from build123d import *

# Parameters (mm, degrees)
BOSS_EXTRUDE1_DEPTH = 6
FILLET1_R           = 10


with BuildPart() as part:
    # Sketch1 → Boss-Extrude1 (new body)
    with BuildSketch(Plane.XY):
        Polygon((0, 0), (24, 0), (24, -3), (34, -3), (34, 0), (154, 0), (154, -3), (164, -3), (164, 0), (193, 0), (179, 10), (29, 10), align=None)
        with BuildLine():
            Line((53.5, 7), (60.5, 7))
            ThreePointArc((60.5, 7), (60.853553391, 6.853553391), (61, 6.5))
            Line((61, 6.5), (61, 3.5))
            ThreePointArc((61, 3.5), (60.853553391, 3.146446609), (60.5, 3))
            Line((60.5, 3), (53.5, 3))
            ThreePointArc((53.5, 3), (53.146446609, 3.146446609), (53, 3.5))
            Line((53, 3.5), (53, 6.5))
            ThreePointArc((53, 6.5), (53.146446609, 6.853553391), (53.5, 7))
        make_face(mode=Mode.SUBTRACT)
        with BuildLine():
            Line((37.5, 7), (44.5, 7))
            ThreePointArc((44.5, 7), (44.853553391, 6.853553391), (45, 6.5))
            Line((45, 6.5), (45, 3.5))
            ThreePointArc((45, 3.5), (44.853553391, 3.146446609), (44.5, 3))
            Line((44.5, 3), (37.5, 3))
            ThreePointArc((37.5, 3), (37.146446609, 3.146446609), (37, 3.5))
            Line((37, 3.5), (37, 6.5))
            ThreePointArc((37, 6.5), (37.146446609, 6.853553391), (37.5, 7))
        make_face(mode=Mode.SUBTRACT)
        with BuildLine():
            Line((69.5, 7), (76.5, 7))
            ThreePointArc((76.5, 7), (76.853553391, 6.853553391), (77, 6.5))
            Line((77, 6.5), (77, 3.5))
            ThreePointArc((77, 3.5), (76.853553391, 3.146446609), (76.5, 3))
            Line((76.5, 3), (69.5, 3))
            ThreePointArc((69.5, 3), (69.146446609, 3.146446609), (69, 3.5))
            Line((69, 3.5), (69, 6.5))
            ThreePointArc((69, 6.5), (69.146446609, 6.853553391), (69.5, 7))
        make_face(mode=Mode.SUBTRACT)
        with BuildLine():
            Line((85.5, 7), (92.5, 7))
            ThreePointArc((92.5, 7), (92.853553391, 6.853553391), (93, 6.5))
            Line((93, 6.5), (93, 3.5))
            ThreePointArc((93, 3.5), (92.853553391, 3.146446609), (92.5, 3))
            Line((92.5, 3), (85.5, 3))
            ThreePointArc((85.5, 3), (85.146446609, 3.146446609), (85, 3.5))
            Line((85, 3.5), (85, 6.5))
            ThreePointArc((85, 6.5), (85.146446609, 6.853553391), (85.5, 7))
        make_face(mode=Mode.SUBTRACT)
        with BuildLine():
            Line((101.5, 7), (108.5, 7))
            ThreePointArc((108.5, 7), (108.853553391, 6.853553391), (109, 6.5))
            Line((109, 6.5), (109, 3.5))
            ThreePointArc((109, 3.5), (108.853553391, 3.146446609), (108.5, 3))
            Line((108.5, 3), (101.5, 3))
            ThreePointArc((101.5, 3), (101.146446609, 3.146446609), (101, 3.5))
            Line((101, 3.5), (101, 6.5))
            ThreePointArc((101, 6.5), (101.146446609, 6.853553391), (101.5, 7))
        make_face(mode=Mode.SUBTRACT)
        with BuildLine():
            Line((117.5, 7), (124.5, 7))
            ThreePointArc((124.5, 7), (124.853553391, 6.853553391), (125, 6.5))
            Line((125, 6.5), (125, 3.5))
            ThreePointArc((125, 3.5), (124.853553391, 3.146446609), (124.5, 3))
            Line((124.5, 3), (117.5, 3))
            ThreePointArc((117.5, 3), (117.146446609, 3.146446609), (117, 3.5))
            Line((117, 3.5), (117, 6.5))
            ThreePointArc((117, 6.5), (117.146446609, 6.853553391), (117.5, 7))
        make_face(mode=Mode.SUBTRACT)
        with BuildLine():
            Line((133.5, 7), (140.5, 7))
            ThreePointArc((140.5, 7), (140.853553391, 6.853553391), (141, 6.5))
            Line((141, 6.5), (141, 3.5))
            ThreePointArc((141, 3.5), (140.853553391, 3.146446609), (140.5, 3))
            Line((140.5, 3), (133.5, 3))
            ThreePointArc((133.5, 3), (133.146446609, 3.146446609), (133, 3.5))
            Line((133, 3.5), (133, 6.5))
            ThreePointArc((133, 6.5), (133.146446609, 6.853553391), (133.5, 7))
        make_face(mode=Mode.SUBTRACT)
        with BuildLine():
            Line((149.5, 7), (156.5, 7))
            ThreePointArc((156.5, 7), (156.853553391, 6.853553391), (157, 6.5))
            Line((157, 6.5), (157, 3.5))
            ThreePointArc((157, 3.5), (156.853553391, 3.146446609), (156.5, 3))
            Line((156.5, 3), (149.5, 3))
            ThreePointArc((149.5, 3), (149.146446609, 3.146446609), (149, 3.5))
            Line((149, 3.5), (149, 6.5))
            ThreePointArc((149, 6.5), (149.146446609, 6.853553391), (149.5, 7))
        make_face(mode=Mode.SUBTRACT)
        with BuildLine():
            Line((165.5, 7), (172.5, 7))
            ThreePointArc((172.5, 7), (172.853553391, 6.853553391), (173, 6.5))
            Line((173, 6.5), (173, 3.5))
            ThreePointArc((173, 3.5), (172.853553391, 3.146446609), (172.5, 3))
            Line((172.5, 3), (165.5, 3))
            ThreePointArc((165.5, 3), (165.146446609, 3.146446609), (165, 3.5))
            Line((165, 3.5), (165, 6.5))
            ThreePointArc((165, 6.5), (165.146446609, 6.853553391), (165.5, 7))
        make_face(mode=Mode.SUBTRACT)
    extrude(amount=BOSS_EXTRUDE1_DEPTH)

    # Fillet1
    fillet1_edges = [part.edges().sort_by_distance(p)[0] for p in [
        (29, 10, 3),
        (179, 10, 3),
    ]]
    fillet(fillet1_edges, radius=FILLET1_R)


solid = part.part
Design review of the part built by this model. Coordinates are the model's own, in mm. A direction names the side the tool comes from. Round coordinates to 2 decimals unless told otherwise and drop trailing zeros. Write each loop counter-clockwise with the first axis right and the second up, starting at its lowest first coordinate (ties: lowest second). Pieces come first, ordered by that corner, then holes.
Item 1: Wall thickness on L1, parallel to X at y = -0.5, z = 4.7; L2, parallel to Y at x = 100.5, z = 0.5; L3, parallel to Y at x = 27.5, z = 2.25: over which ranges is each line inside the solid? List them lowest first.
Item 2: For faces 1 (the flat face through (57, 7, 3)), 2 (the flat face through (164, -2, 3)), 3 (the flat face through (159, -3, 3)), 4 (the flat face through (154, -1, 3)), 5 (the flat face through (13.9, 4.793, 2.958)), list the 3-axis set-ups (+Z, -Z, +X, -X, +Y, -Y) from which the entire face can be reached by the end or side of a thin tool; tool diameter is ignored.
Item 3: For pin 1 Ø3 at (x, z) = (131.5, 2) entering from -Y; pin 2 Ø3.5 at (y, z) = (-1, 4.5) entering from +X; pin 3 Ø3.5 at (y, z) = (4.5, 3) entering from +X, all flat-tipped, find the tip position at first contact; note any pin that passes through.
Item 4: Consider section C-C on x = 99. Give the boundary of the cut face in (y, z), and give its area (3 significant figures).
Item 5: Consider section A-A on x = 152. Give the boundary of the cut face in (y, z).
Item 6: Consider section B-B on z = 1.6. Count the separate pieces of the cut face and the enclosed holes in it, and give its area (3 significant figures).
Item 7: Draft analysis for pull direction X (two halves, no side actions). For faces 6 (the flat face through (95, 5, 0)), 7 (the flat face through (169, 7, 3)), 8 (the flat face through (24, -1, 3)), state which applies: released by +X, released by -X, zero draft, split by the parting line, or undercut.
Check values:
1. L1: x = 24 to 34, 154 to 164
1. L2: y = 0 to 10
1. L3: y = -3 to 9.48
2. face 1: +Z, -Z
2. face 2: +Z, -Z, +X, -Y
2. face 3: +Z, -Z, +X, -X, -Y
2. face 4: +Z, -Z, -Y
2. face 5: +Z, -Z, -X, +Y
3. pin 1: stops at y = 0
3. pin 2: stops at x = 193
3. pin 3: stops at x = 189.15
4. outline: (0, 0) - (10, 0) - (10, 6) - (0, 6) - close
4. area: 60.0 mm2
5. outline: (0, 0) - (3, 0) - (3, 6) - (0, 6) - close; (7, 0) - (10, 0) - (10, 6) - (7, 6) - close
6. separate pieces: 1
6. enclosed holes: 9
6. area: 1,490 mm2
7. face 6: zero draft
7. face 7: undercut
7. face 8: released by -X
